Geometry: final body of the model. Coordinates: model frame, mm. A direction names the side the tool comes from. Coordinates: 2 decimals unless noted, no trailing zeros. Write each loop counter-clockwise with the first axis right and the second up, starting at its lowest first coordinate (ties: lowest second). Pieces come first, ordered by that corner, then holes. Notation, with made-up numbers: (-35.75, -30) - (18.25, -30) arc R37 ccw to (18.25, 9) - close; hole circle Ø11 at (-2.75, 23). An arc over 180 degrees is marked (long way). Put each result on its own line as item: value.
```python
from build123d import *

# Parameters (mm, degrees)
F0_R     = 9.525
F1_DEPTH = 7.62
F2_R     = 12.7
F3_DEPTH = 7.9502
F5_R     = 2.54


# Not quite as in the source:
# - a fillet or chamfer that OpenCascade refuses, or shapes differently, is made with other operations: its cross-section is extruded or revolved along the edge and cut away or added


with BuildPart() as f1:
    # F0 (on Front) → F1 (new body)
    with BuildSketch(Plane.XZ):
        Circle(F0_R)
    extrude(amount=F1_DEPTH)

    # F2 (on face) → F3 (join)
    with BuildSketch(Plane.XZ.offset(7.62)):
        Circle(F2_R)
    extrude(amount=F3_DEPTH)

    # F4: fillet of radius 4.0132 on 2 edges, made by hand

    # F4_s1 → F4_t2 (revolve, cut)
    with BuildSketch(Plane.XY):
        with BuildLine():
            ThreePointArc((12.7, -11.557), (11.5245609343, -14.3947609343), (8.6868, -15.5702))
            Line((8.6868, -15.5702), (12.7, -15.5702))
            Line((12.7, -15.5702), (12.7, -11.557))
        make_face()
    revolve(axis=Axis((0, -15.5702, 0), (0, -1, 0)), mode=Mode.SUBTRACT)

    # F4_s3 → F4_t4 (revolve, cut)
    with BuildSketch(Plane.XY):
        with BuildLine():
            ThreePointArc((12.7, -11.5446904337), (11.8068671852, -9.0206153555), (9.525, -7.62))
            Line((9.525, -7.62), (12.7, -7.62))
            Line((12.7, -7.62), (12.7, -11.5446904337))
        make_face()
    revolve(axis=Axis((0, -7.62, 0), (0, -1, 0)), mode=Mode.SUBTRACT)

    # F5
    f5_edges = [f1.edges().sort_by_distance(p)[0] for p in [
        (-9.525, 0, 0),
    ]]
    fillet(f5_edges, radius=F5_R)


solid = f1.part
```
1. Section query A-A (x = 0). Return loops of the section in (y, z) (3 decimals), then the cut area to 3 significant figures.
Answer below:
outline: (-15.57, -8.687) arc R4.013 ccw to (-11.557, -12.7) - (-11.545, -12.7) arc R4.013 ccw to (-7.62, -9.525) - (-2.54, -9.525) arc R2.54 ccw to (0, -6.985) - (0, 6.985) arc R2.54 ccw to (-2.54, 9.525) - (-7.62, 9.525) arc R4.013 ccw to (-11.545, 12.7) - (-11.557, 12.7) arc R4.013 ccw to (-15.57, 8.687) - close
area: 331 mm²
2. Section query B-B (z = 0). Return loops of the section in (x, y) (3 decimals).
Answer below:
outline: (-12.7, -11.557) arc R4.013 ccw to (-8.687, -15.57) - (8.687, -15.57) arc R4.013 ccw to (12.7, -11.557) - (12.7, -11.545) arc R4.013 ccw to (9.525, -7.62) - (9.525, -2.54) arc R2.54 ccw to (6.985, 0) - (-6.985, 0) arc R2.54 ccw to (-9.525, -2.54) - (-9.525, -7.62) arc R4.013 ccw to (-12.7, -11.545) - close
3. Ray query, probe 1 along Z at (x, y) = (2.25, -4.75); probe 2 along Y at (x, z) = (-1, 10.75); probe 3 along X at (y, z) = (-9.25, 2.5). Return the intervals inside material, ascending. Write a range as from..to.
Answer below:
probe 1: z = -9.26..9.26
probe 2: y = -14.97..-8.13
probe 3: x = -11.72..11.72
4. Set-up query: faces 1 (the flat face through (0, 0, 0)), 2 (the cylindrical face through (-7.559, -5.044, -5.796)). Return all of +Z, -Z, +X, -X, +Y, -Y with unobstructed straight access to the full face (end or side cutting, diameter ignored); none if empty.
Answer below:
face 1: +Z, -Z, +X, -X, +Y
face 2: +Y
5. Section query D-D (y = -12.5). Return loops of the section in (x, z), then the cut area to 3 significant figures.
Answer below:
outline: circle Ø25.18 at (0, 0)
area: 498 mm²
6. Section query C-C (y = -4.5). Return loops of the section in (x, z) (3 decimals), then the cut area to 3 significant figures.
Answer below:
outline: circle Ø19.05 at (0, 0)
area: 285 mm²
7. Pin query (flat end, axial travel): pin 1 Ø5 at (y, z) = (-3, -9) entering from -X; pin 2 Ø1 at (x, y) = (-3, -6.5) entering from -Z; pin 3 Ø1.5 at (x, y) = (4, -10.5) entering from +Z. Return the tip coordinate at first contact, or that it passes through.
Answer below:
pin 1: stops at x = -6.96
pin 2: stops at z = -9.19
pin 3: stops at z = 12.19
